```python
from build123d import *

# Parameters (mm, degrees)
SKETCH2_R           = 2.4892
SKETCH2_R_2         = 12.7
BOSS_EXTRUDE1_DEPTH = 2.286
FILLET6_R           = 12.7
FILLET7_R           = 15.24


with BuildPart() as part:
    # Sketch2 → Boss-Extrude1 (new body)
    with BuildSketch(Plane.XY):
        Polygon((33.430156219, 560.153270419), (33.430156219, 610.953270419), (-17.369843781, 610.953270419), (-70.882869838, 630.430419049), (-92.601148921, 570.759937623), (-96.944804742, 558.825841339), (-49.208419606, 541.451218058), (-17.464279743, 534.753270419), (33.335720257, 534.753270419), (33.335720257, 547.453270419), align=None)
        with Locations((-4.764279743, 566.503270419)):
            Circle(SKETCH2_R, mode=Mode.SUBTRACT)
        with Locations((-4.764279743, 579.203270419)):
            Circle(SKETCH2_R, mode=Mode.SUBTRACT)
        with Locations((7.935720257, 566.503270419)):
            Circle(SKETCH2_R, mode=Mode.SUBTRACT)
        with Locations((20.635720257, 566.503270419)):
            Circle(SKETCH2_R, mode=Mode.SUBTRACT)
        with Locations((7.935720257, 579.203270419)):
            Circle(SKETCH2_R, mode=Mode.SUBTRACT)
        with Locations((20.635720257, 579.203270419)):
            Circle(SKETCH2_R, mode=Mode.SUBTRACT)
        with Locations((-4.764279743, 591.903270419)):
            Circle(SKETCH2_R, mode=Mode.SUBTRACT)
        with Locations((-4.764279743, 604.603270419)):
            Circle(SKETCH2_R, mode=Mode.SUBTRACT)
        with Locations((7.935720257, 591.903270419)):
            Circle(SKETCH2_R, mode=Mode.SUBTRACT)
        with Locations((20.635720257, 591.903270419)):
            Circle(SKETCH2_R, mode=Mode.SUBTRACT)
        with Locations((7.935720257, 604.603270419)):
            Circle(SKETCH2_R, mode=Mode.SUBTRACT)
        with Locations((20.635720257, 604.603270419)):
            Circle(SKETCH2_R, mode=Mode.SUBTRACT)
        with Locations((20.635720257, 553.803270419)):
            Circle(SKETCH2_R, mode=Mode.SUBTRACT)
        with Locations((-4.764279743, 553.803270419)):
            Circle(SKETCH2_R, mode=Mode.SUBTRACT)
        with Locations((7.935720257, 553.803270419)):
            Circle(SKETCH2_R, mode=Mode.SUBTRACT)
        with Locations((20.635720257, 541.103270419)):
            Circle(SKETCH2_R, mode=Mode.SUBTRACT)
        with Locations((7.935720257, 541.103270419)):
            Circle(SKETCH2_R, mode=Mode.SUBTRACT)
        with Locations((-4.764279743, 541.103270419)):
            Circle(SKETCH2_R, mode=Mode.SUBTRACT)
        with Locations((-37.25240889, 611.432403444)):
            Circle(SKETCH2_R, mode=Mode.SUBTRACT)
        with Locations((-50.283376351, 575.630114592)):
            Circle(SKETCH2_R, mode=Mode.SUBTRACT)
        with Locations((-62.217472635, 579.973770413)):
            Circle(SKETCH2_R, mode=Mode.SUBTRACT)
        with Locations((-74.151568919, 584.317426233)):
            Circle(SKETCH2_R, mode=Mode.SUBTRACT)
        with Locations((-55.562991918, 598.25680592)):
            Circle(SKETCH2_R_2, mode=Mode.SUBTRACT)
        with Locations((-61.120601458, 620.119715085)):
            Circle(SKETCH2_R, mode=Mode.SUBTRACT)
        with Locations((-49.186505174, 615.776059265)):
            Circle(SKETCH2_R, mode=Mode.SUBTRACT)
        with Locations((-78.495224739, 572.383329949)):
            Circle(SKETCH2_R, mode=Mode.SUBTRACT)
        with Locations((-54.627032171, 563.696018308)):
            Circle(SKETCH2_R, mode=Mode.SUBTRACT)
        with Locations((-66.561128455, 568.039674129)):
            Circle(SKETCH2_R, mode=Mode.SUBTRACT)
        with Locations((-58.970687991, 551.761922025)):
            Circle(SKETCH2_R, mode=Mode.SUBTRACT)
        with Locations((-82.838880559, 560.449233665)):
            Circle(SKETCH2_R, mode=Mode.SUBTRACT)
        with Locations((-70.904784275, 556.105577845)):
            Circle(SKETCH2_R, mode=Mode.SUBTRACT)
    extrude(amount=BOSS_EXTRUDE1_DEPTH)

    # Fillet6
    fillet6_edges = [part.edges().sort_by_distance(p)[0] for p in [
        (-70.882869838, 630.430419049, 1.143),
        (-96.944804742, 558.825841339, 1.143),
        (33.430156219, 610.953270419, 1.143),
        (33.335720257, 534.753270419, 1.143),
    ]]
    fillet(fillet6_edges, radius=FILLET6_R - 0.0001)  # a hair under: the kernel refuses the full size

    # Fillet7
    fillet7_edges = [part.edges().sort_by_distance(p)[0] for p in [
        (-17.464279743, 534.753270419, 1.143),
        (-49.208419606, 541.451218058, 1.143),
        (-17.369843781, 610.953270419, 1.143),
    ]]
    fillet(fillet7_edges, radius=FILLET7_R)


solid = part.part
```
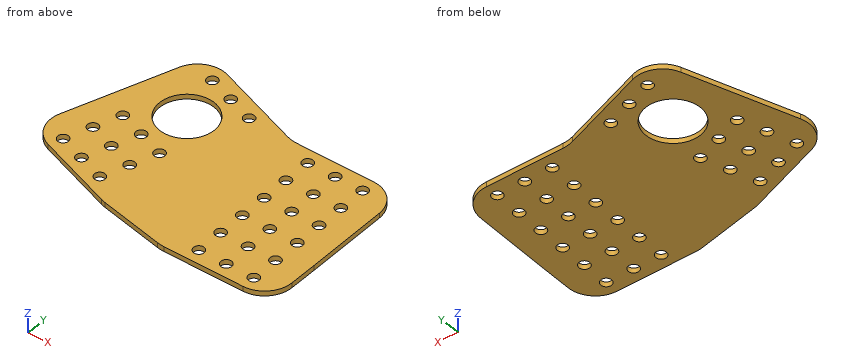
Here's how the part is built. I have some questions about the finished solid (model axes, mm). Round coordinates to 2 decimals unless told otherwise and drop trailing zeros. Order: outer loops, then holes, each group sorted by start corner. A loop starts at its lowest first (then second) coordinate and runs counter-clockwise, first axis right, second up. Notation, with made-up numbers: M -20.75,-33 L 28.25,-33 A7 ccw 28.25,-26 Z; hole C 60,88 d9. An arc over 180 degrees is marked long. One line per question, with ' | ' between items.
1) I want a section at A-A, the plane x = -44.5. Write out the boundary of the cut face in (y, z), then the cut area to 3 significant figures.
Working result:
outline: M 540.46,0 L 592.02,0 L 592.02,2.29 L 540.46,2.29 Z; M 604.49,0 L 620.83,0 L 620.83,2.29 L 604.49,2.29 Z | area: 155 mm²
2) I want a section at B-B, the plane z = 1.75. State how many separate pieces and enclosed holes the cut face has, then the cut area to 3 significant figures.
Working result:
separate pieces: 1 | enclosed holes: 31 | area: 7,960 mm²
3) I need wall thicknesses on line 1 along Y through (x, z) = (-48, 0.65); line 2 along X through (y, z) = (555, 0.4); line 3 along Y through (x, z) = (-54.5, 2.15). Which ranges of each line are inside material? Lowest first, please.
Working result:
line 1: 541.2 to 574.64, 576.62 to 588.05, 608.46 to 613.59, 617.96 to 622.1 | line 2: -86.23 to -73.13, -68.67 to -6.95, -2.58 to 5.75, 10.12 to 18.45, 22.82 to 33.39 | line 3: 543.38 to 561.21, 566.18 to 585.6, 610.91 to 624.47
4) For pin 1 Ø1 at (y, z) = (564, 2) entering from -X, with a flat end and sliding along its axis, tell me the tip position at first contact or that it passes through.
Working result:
pin 1: x = -93.22
